Autodesk Inventor part; units mm, degrees
ref_plane "Work Plane1" through (-12.5, 4.5, 15) normal (0, 1, 0) x (1, 0, 0)
ref_plane "Work Plane2" through (-12.5, -2.5, 15) normal (0, 1, 0) x (1, 0, 0)
ref_plane "Work Plane3" through (-12.5, -7.5, -11) normal (0, -1, 0) x (1, 0, 0)
sketch "Sketch1" plane through (0, 0, 0) normal (1, 0, 0) x (0, 1, 0)
  line L0 (-12.5, 15) -> (12.5, 15)
  line L1 (12.5, 15) -> (12.5, -15)
  line L2 (12.5, -15) -> (-12.5, -15)
  line L3 (-12.5, -15) -> (-12.5, 15)
  line L4 (-12.5, 15) -> (12.5, -15) construction
  line L5 (12.5, 15) -> (-12.5, -15) construction
  point P0 (0, 0)
  dimension "d0" = 30
  dimension "d1" = 25
extrude "Extrusion1" add sketch "Sketch1" along normal mid plane 25
sketch "Sketch5" plane through (-12.5, 12.5, 15) normal (0, 1, 0) x (1, 0, 0)
  line L0 (0, 30) -> (0, 0)
  line L1 (25, 0) -> (25, 30)
  circle A0 centre (12.5, 10) radius 2.65
  line L2 (12.5, 10) -> (12.5, 0) construction
  line L3 (0, 0) -> (25, 0)
  point P0 (12.5, 15)
  dimension "d22" = 5.3
  dimension "d25" = 10
extrude "Extrusion5" cut sketch "Sketch5" against normal through all
ref_plane "Work Plane1" through (-12.5, 4.5, 15) normal (0, 1, 0) x (1, 0, 0)
sketch "Sketch2" plane through (-12.5, 4.5, 15) normal (0, 1, 0) x (1, 0, 0)
  circle A0 centre (12.5, 26) radius 9 construction
  circle A1 centre (12.5, 26) radius 1.75 construction
  line L0 (0, 30) -> (25, 30) construction
  line L1 (12.5, 30) -> (12.5, 26)
  circle A2 centre (12.5, 26) radius 10
  point P0 (12.5, 15)
  dimension "d5" = 4
  dimension "d6" = 3.5
  dimension "d7" = 18
  dimension "d8" = 1
extrude "Extrusion2" cut sketch "Sketch2" against normal mid plane 11
sketch "Sketch3" plane through (-12.5, 4.5, 15) normal (0, 1, 0) x (1, 0, 0)
  arc A0 (3.3348, 30) -> (21.6652, 30) centre (12.5, 26) ccw
  circle A1 centre (12.5, 26) radius 2.25
  point P0 (12.5, 15)
  point P1 (20, 16)
  point P2 (0, 16)
  dimension "d11" = 4.5
extrude "Extrusion3" cut sketch "Sketch3" along normal blind 10 and the other way blind 16
ref_plane "Work Plane2" through (-12.5, -2.5, 15) normal (0, 1, 0) x (1, 0, 0)
sketch "Sketch4" plane through (-12.5, -2.5, 15) normal (0, 1, 0) x (1, 0, 0)
  circle A0 centre (12.5, 26) radius 2.25
  line L0 (12.5, 30.2147) -> (16.15, 28.1073) construction
  line L1 (16.15, 28.1073) -> (16.15, 23.8927)
  line L2 (16.15, 23.8927) -> (12.5, 21.7853)
  line L3 (12.5, 21.7853) -> (8.85, 23.8927)
  line L4 (8.85, 23.8927) -> (8.85, 28.1073)
  line L5 (8.85, 28.1073) -> (12.5, 30.2147) construction
  line L6 (8.85, 28.1073) -> (8.85, 36.3706)
  line L7 (8.85, 36.3706) -> (16.15, 36.3706)
  line L8 (16.15, 36.3706) -> (16.15, 28.1073)
  point P0 (12.5, 15)
  dimension "d46" = 7.3
extrude "Extrusion4" cut sketch "Sketch4" against normal blind 3.5
fillet "Fillet1" radius 2 2 edges at (9.1652, 4.5, -15) (-9.1652, 4.5, -15)
fillet "Fillet1" radius 4 4 edges at (12.5, 0, -15) (-12.5, 0, -15) (-12.5, 0, 15) (12.5, 0, 15)
fillet "Fillet1" radius 2 4 edges at (12.5, 12.5, 0) (0, 12.5, 15) (-12.5, 12.5, 0) (0, 12.5, -15)
ref_plane "Work Plane3" through (-12.5, -7.5, -11) normal (0, -1, 0) x (1, 0, 0)
sketch "Sketch6" plane through (-12.5, -7.5, -11) normal (0, -1, 0) x (1, 0, 0)
  circle A0 centre (12.5, 16) radius 2.65
  circle A1 centre (12.5, 16) radius 4.5
  point P0 (12.5, 11)
  dimension "d27" = 9
extrude "Extrusion6" cut sketch "Sketch6" against normal through all contours A0 | A1
sketch "Sketch9" plane through (0, 0, 0) normal (1, 0, 0) x (0, 1, 0)
  line L0 (-17.5, -11) -> (17.5, -11)
  line L1 (-1, -8.75) -> (-1, -13.25)
  line L2 (10, -13.25) -> (10, -8.75)
  line L3 (10, -13.25) -> (10, -14.75)
  line L4 (10, -14.75) -> (9.5, -14.25)
  line L5 (9.5, -14.25) -> (9.5, -13.25)
  line L6 (9.5, -13.25) -> (10, -13.25)
  line L7 (-1, -13.25) -> (-0.5, -13.25)
  line L8 (-0.5, -13.25) -> (-0.5, -14.25)
  line L9 (-0.5, -14.25) -> (-1, -14.75)
  line L10 (-1, -14.75) -> (-1, -13.25)
  point P0 (0, 0)
  dimension "d38" = 0.5
  dimension "d39" = 1
  dimension "d40" = 45
  dimension "d41" = 0.5
  dimension "d42" = 1
  dimension "d43" = 45
revolve "Revolution1" add sketch "Sketch9" angle 360 about axis through (0, 4.5, -11) along (0, 1, 0)
properties part number "YIdler"
Input: part model. Units: mm. Frame: model coordinates. A direction names the side the tool comes from. Round coordinates to 2 decimals unless told otherwise and drop trailing zeros. Loops run counter-clockwise (first coordinate to the right, second up) from the corner with the lowest first, then second, coordinate; pieces in that order, holes last. Notation, with made-up numbers: (-6.5, -26) -> (45.5, -26) arc R15 ccw to (45.5, -13) -> close; hole circle Ø2 at (-33, 32.5). An arc over 180 degrees is marked (long way). Answer as a JSON object with one key per item and string values. Group by question number.
1) Section query C-C on y = 3.75. Output: boundary loops of the cut face in (x, z), plus the area to 3 significant figures.
2) Section query B-B on y = -3.5. Output: boundary loops of the cut face in (x, z), plus the area to 3 significant figures.
3) Section query A-A on z = 5. Output: boundary loops of the cut face in (x, y), plus the area to 3 significant figures.
4) Pin query (flat end, axial travel): pin 1 (2.5 mm diameter, centred on x = 0, z = -11, fed in from +Y); pin 2 (3 mm diameter, centred on y = -3.5, z = -12.5, fed in from +X); pin 3 (3 mm diameter, centred on x = -0.5, z = 5, fed in from -Y); pin 4 (8.5 mm diameter, centred on x = 0, z = 5, fed in from +Y). Return the tip coordinate at first contact, or that it passes through.
5) Reachability of faces 1 (the cylindrical face through (11.8, -0.84, -13.26)), 2 (the flat face through (0, -11.5, -11)), 3 (the flat face through (-1.799, -4.226, -7.824)), 4 (the cylindrical face through (0, 5, -1)), 5 (the flat face through (12.5, -1, 0)) from +Z, -Z, +X, -X, +Y, -Y: full face, straight path, thin tool, end or side. Return the list, or none.
6) Ray query, L1, parallel to Z at x = 0, y = -11; L2, parallel to Y at x = -4.75, z = -3.5; L3, parallel to Y at x = 1.25, z = -13.5. Return the intervals inside material, ascending.
7) Section query D-D on x = -6.25. Output: boundary loops of the cut face in (y, z), plus the area to 3 significant figures.
8) Draft query along Y for faces 6 (the cylindrical face through (9.936, 4.423, -13.637)), 7 (the cylindrical face through (-0.98, 2.36, 0.61)), 8 (the cylindrical face through (-11.9, 11.93, 0.15)). Return one class per face: +Y half, -Y half, draft (parallel to the pull), parting line (faces both ways), or undercut.
Reply:
{
 "1": {"outline": "(-12.5, -11) arc R4 ccw to (-10.48, -14.47) arc R2 ccw to (-9.86, -12.67) arc R10 cw (long way) to (9.86, -12.67) arc R2 ccw to (10.48, -14.47) arc R4 ccw to (12.5, -11) -> (12.5, 11) arc R4 ccw to (8.5, 15) -> (-8.5, 15) arc R4 ccw to (-12.5, 11) -> close; hole circle Ø9 at (0, 5)", "area": "436 mm2"},
 "2": {"outline": "(-12.5, -11) arc R4 ccw to (-8.5, -15) -> (-3.65, -15) -> (-3.65, -8.89) -> (0, -6.79) -> (3.65, -8.89) -> (3.65, -15) -> (8.5, -15) arc R4 ccw to (12.5, -11) -> (12.5, 11) arc R4 ccw to (8.5, 15) -> (-8.5, 15) arc R4 ccw to (-12.5, 11) -> close; hole circle Ø9 at (0, 5)", "area": "620 mm2"},
 "3": {"outline": "(-12.5, -12.5) -> (-2.65, -12.5) -> (-2.65, -7.5) -> (-4.5, -7.5) -> (-4.5, 12.5) -> (-10.5, 12.5) arc R2 ccw to (-12.5, 10.5) -> close; (2.65, -12.5) -> (12.5, -12.5) -> (12.5, 10.5) arc R2 ccw to (10.5, 12.5) -> (4.5, 12.5) -> (4.5, -7.5) -> (2.65, -7.5) -> close", "area": "417 mm2"},
 "4": {"pin 1": "stops at y = -11.5", "pin 2": "stops at x = 12.5", "pin 3": "passes through", "pin 4": "stops at y = -7.5"},
 "5": {"face 1": "-Z, +X, +Y, -Y", "face 2": "+Y", "face 3": "-Z", "face 4": "none", "face 5": "+Z, -Z, +X, +Y, -Y"},
 "6": {"L1": "z = -15 to -13.25, -8.75 to 2.35, 7.65 to 15", "L2": "y = -12.5 to -1, 10 to 12.5", "L3": "y = -12.5 to -6, -2.5 to -0.5, 9.5 to 12.44"},
 "7": {"outline": "(-12.5, -15) -> (-1, -15) -> (-1, -3.19) -> (10, -3.19) -> (10, -15) -> (10.5, -15) arc R2 ccw to (12.5, -13) -> (12.5, 13) arc R2 ccw to (10.5, 15) -> (-12.5, 15) -> close", "area": "618 mm2"},
 "8": {"face 6": "undercut", "face 7": "draft", "face 8": "+Y half"}
}
